```python
from build123d import *

# Parameters (mm, degrees)
CORTAR_EXTRUIR4_DEPTH      = 1
CROQUIS7_R                 = 7.5
CORTAR_EXTRUIR5_DEPTH      = 9
CORTAR_EXTRUIR6_DEPTH      = 9
CORTAR_EXTRUIR8_DEPTH      = 5
CORTAR_EXTRUIR8_DEPTH_BACK = 35.470929781
CROQUIS10_R                = 3
CROQUIS11_R                = 1.5
CORTAR_EXTRUIR9_DEPTH      = 5.2
CROQUIS12_W                = 21.5
CROQUIS12_H                = 4.5


with BuildPart() as part:
    # Croquis1 → Revolución1 (revolve)
    with BuildSketch(Plane(origin=(0, 0, 0), x_dir=(0, 0, -1), z_dir=(1, 0, 0))):
        Polygon((0, 0), (6.15, 0), (6.15, 14.5), (-15.35, 14.5), (-15.35, 15.2), (-16.05, 15.2), (-16.05, 0), align=None)
    revolve(axis=Axis((0, 0, 0), (0, 0, 1)))

    # Croquis5 → Cortar-Extruir4 (cut)
    with BuildSketch(Plane.XY.offset(16.05)):
        with BuildLine():
            ThreePointArc((-1.4, 4.276680956), (0, 4.5), (1.4, 4.276680956))
            Line((1.4, 4.276680956), (5.9, 11.487783507))
            ThreePointArc((5.9, 11.487783507), (0, 13.2), (-5.9, 11.487783507))
            Line((-5.9, 11.487783507), (-1.4, 4.276680956))
        make_face()
        with BuildLine():
            Line((6.99871235, 10.853441636), (3.003714352, 3.350776043))
            ThreePointArc((3.003714352, 3.350776043), (3.897114317, 2.25), (4.403714352, 0.925904913))
            Line((4.403714352, 0.925904913), (12.89871235, 0.634341871))
            ThreePointArc((12.89871235, 0.634341871), (11.43153533, 6.6), (6.99871235, 10.853441636))
        make_face()
        with BuildLine():
            Line((12.89871235, -0.634341871), (4.403714352, -0.925904913))
            ThreePointArc((4.403714352, -0.925904913), (3.897114317, -2.25), (3.003714352, -3.350776043))
            Line((3.003714352, -3.350776043), (6.99871235, -10.853441636))
            ThreePointArc((6.99871235, -10.853441636), (11.43153533, -6.6), (12.89871235, -0.634341871))
        make_face()
        with BuildLine():
            Line((5.9, -11.487783507), (1.4, -4.276680956))
            ThreePointArc((1.4, -4.276680956), (0, -4.5), (-1.4, -4.276680956))
            Line((-1.4, -4.276680956), (-5.9, -11.487783507))
            ThreePointArc((-5.9, -11.487783507), (0, -13.2), (5.9, -11.487783507))
        make_face()
        with BuildLine():
            ThreePointArc((-3.003714352, -3.350776043), (-3.897114317, -2.25), (-4.403714352, -0.925904913))
            Line((-4.403714352, -0.925904913), (-12.89871235, -0.634341871))
            ThreePointArc((-12.89871235, -0.634341871), (-11.43153533, -6.6), (-6.99871235, -10.853441636))
            Line((-6.99871235, -10.853441636), (-3.003714352, -3.350776043))
        make_face()
        with BuildLine():
            ThreePointArc((-4.403714352, 0.925904913), (-3.897114317, 2.25), (-3.003714352, 3.350776043))
            Line((-3.003714352, 3.350776043), (-6.99871235, 10.853441636))
            ThreePointArc((-6.99871235, 10.853441636), (-11.43153533, 6.6), (-12.89871235, 0.634341871))
            Line((-12.89871235, 0.634341871), (-4.403714352, 0.925904913))
        make_face()
    extrude(amount=-CORTAR_EXTRUIR4_DEPTH, mode=Mode.SUBTRACT)

    # Croquis7 → Cortar-Extruir5 (cut)
    with BuildSketch(Plane(origin=(0, 0, -6.15), x_dir=(-1, 0, 0), z_dir=(0, 0, -1))):
        with Locations(Location((0, 0, 0), (0, 0, 90))):
            Circle(CROQUIS7_R)
    extrude(amount=-CORTAR_EXTRUIR5_DEPTH, mode=Mode.SUBTRACT)

    # Croquis8 → Cortar-Extruir6 (cut)
    with BuildSketch(Plane(origin=(0, 0, 2.85), x_dir=(-1, 0, 0), z_dir=(0, 0, -1))):
        with BuildLine():
            Line((-1.140175425, -1.05), (1.140175425, -1.05))
            ThreePointArc((1.140175425, -1.05), (0, 1.55), (-1.140175425, -1.05))
        make_face()
    extrude(amount=-CORTAR_EXTRUIR6_DEPTH, mode=Mode.SUBTRACT)

    # Croquis10 → Cortar-Extruir8 (cut, two sides: drawn at the far end of the back side and taken through both)
    with BuildSketch(Plane(origin=(0, -11.25, 0), x_dir=(1, 0, 0), z_dir=(0, 1, 0)).offset(-CORTAR_EXTRUIR8_DEPTH_BACK)):
        with Locations(Location((0, -8.85, 0), (0, 0, 270))):
            Circle(CROQUIS10_R)
    extrude(amount=CORTAR_EXTRUIR8_DEPTH + CORTAR_EXTRUIR8_DEPTH_BACK, mode=Mode.SUBTRACT)

    # Croquis11 → Cortar-Extruir9 (cut)
    with BuildSketch(Plane.XZ.offset(6.25)):
        with Locations(Location((0, 8.85, 0), (0, 0, 270))):
            Circle(CROQUIS11_R)
    extrude(amount=-CORTAR_EXTRUIR9_DEPTH, mode=Mode.SUBTRACT)

    # Croquis12 → Revolución2 (revolve)
    with BuildSketch(Plane(origin=(0, 0, 0), x_dir=(0, 0, -1), z_dir=(1, 0, 0)), mode=Mode.PRIVATE) as revoluci_n2_sk:
        with Locations((-4.6, 16.75)):
            Rectangle(CROQUIS12_W, CROQUIS12_H)
    revolve(revoluci_n2_sk.sketch.rotate(Axis((0, 0, 12.043120257), (0, 0, -1)), 90), axis=Axis((0, 0, 12.043120257), (0, 0, -1)))


solid = part.part
```
The listing builds one solid part. Answer for the finished solid, in the listing's coordinates (mm). A direction names the side the tool comes from. Give positions to 0.01 mm unless a question says otherwise; leave off trailing zeros. Loops run counter-clockwise (first coordinate to the right, second up) from the corner with the lowest first, then second, coordinate; pieces in that order, holes last. Notation, with made-up numbers: (75, -35.75) - (89, -35.75) arc R14 cw to (89, -20.75) - close; hole circle Ø4 at (55.5, -4.5). An arc over 180 degrees is marked (long way). Answer as CSV lines item,"result". Start each with the question number.
Item 1: Find the intervals of material crossed by line 1 (Y direction, x = 1, z = 6.5); line 2 (Y direction, x = 0, z = 9.5); line 3 (Z direction, x = 3, y = 11), in increasing order. Write a range as from..to.
Item 2: The mould has two halves that part along X. Classify faces 1 (the face through (0, 2, 2.85)), 2 (the face through (0, 0, 16.05)): +X half, -X half, draft (parallel to the pull), parting line (faces both ways), or undercut.
Item 3: For faces 3 (the face through (9, -13, 15.35)), 4 (the face through (0.33, -7.493, -1.713)), 5 (the face through (-8, 0, -6.15)), 6 (the face through (0, -14.5, 8.8)), determine the directions among +Z, -Z, +X, -X, +Y, -Y from which every point of the face is accessible in a straight line to the end or side of a thin tool.
Item 4: A cutting plane is placed at A-A on z = 8.85. Determine the outline of the cut face in (x, y).
Item 5: A cutting plane is placed at B-B on y = -8. Determine the outline of the cut face in (x, z).
Item 6: A cutting plane is placed at D-D on y = 0. Determine the outline of the cut face in (x, z), then the cut area to 3 significant figures.
Item 7: Each of these flat-tipped pins is pushed along its axis until it touches: pin 1 (5.5 mm diameter, centred on x = 0, z = 8.85, fed in from +Y); pin 2 (6 mm diameter, centred on y = 6, z = 7.5, fed in from -X); pin 3 (5 mm diameter, centred on x = -0.5, z = 9.5, fed in from -Y). Where does it stop, or does it pass through?
Found:
1,line 1,"y = -18.97..-14.47, -6.25..-1.05, 1.18..18.97"
1,line 2,"y = -19..-14.5, 1.55..19"
1,line 3,"z = -6.15..15.05"
2,face 1,"undercut"
2,face 2,"draft"
3,face 3,"+Z"
3,face 4,"-Z"
3,face 5,"-Z, +X, -X, +Y, -Y"
3,face 6,"none"
4,outline,"circle Ø38 at (0, 0); hole (-3, -14.19) arc R14.5 ccw to (3, -14.19) - (3, -6.25) - (1.5, -6.25) - (1.5, -1.05) - (1.14, -1.05) arc R1.55 ccw (long way) to (-1.14, -1.05) - (-1.5, -1.05) - (-1.5, -6.25) - (-3, -6.25) - close"
5,outline,"(-17.23, -6.15) - (17.23, -6.15) - (17.23, 15.35) - (12.92, 15.35) - (12.92, 16.05) - (10.47, 16.05) - (10.47, 15.05) - (5.48, 15.05) - (5.48, 16.05) - (3.72, 16.05) - (3.72, 15.05) - (-3.72, 15.05) - (-3.72, 16.05) - (-5.48, 16.05) - (-5.48, 15.05) - (-10.47, 15.05) - (-10.47, 16.05) - (-12.92, 16.05) - (-12.92, 15.35) - (-17.23, 15.35) - close; hole circle Ø6 at (0, 8.85)"
6,outline,"(-19, -6.15) - (-7.5, -6.15) - (-7.5, 2.85) - (-1.55, 2.85) - (-1.55, 11.85) - (1.55, 11.85) - (1.55, 2.85) - (7.5, 2.85) - (7.5, -6.15) - (19, -6.15) - (19, 15.35) - (15.2, 15.35) - (15.2, 16.05) - (-15.2, 16.05) - (-15.2, 15.35) - (-19, 15.35) - close"
6,area,"675 mm^2"
7,pin 1,"stops at y = 19"
7,pin 2,"stops at x = -18.76"
7,pin 3,"stops at y = -19"
